```python
from build123d import *

# Parameters (mm, degrees)
CLIP_DEPTH        = 20.32
BACK_DEPTH        = 40.64
HOLE_DEPTH        = 6.08
COUNTERBORE_DEPTH = 1.397
CHAMFER1_SIZE     = 1.27
CHAMFER2_SIZE     = 0.508


with BuildPart() as part:
    # Sketch1 → clip (new body)
    with BuildSketch(Plane.XY):
        with BuildLine():
            Line((-2.629601498, -9.813806395), (-1.80785103, -6.746991897))
            ThreePointArc((-1.80785103, -6.746991897), (0, 6.985), (1.80785103, -6.746991897))
            Line((1.80785103, -6.746991897), (2.629601498, -9.813806395))
            Line((2.629601498, -9.813806395), (5.929158287, -11.718806395))
            Line((5.929158287, -11.718806395), (7.453158287, -9.079160964))
            Line((7.453158287, -9.079160964), (5.96856706, -8.22203182))
            ThreePointArc((5.96856706, -8.22203182), (9.051691591, -4.614377459), (10.16, 0))
            Line((10.16, 0), (10.16, 12.7))
            Line((10.16, 12.7), (-10.16, 12.7))
            Line((-10.16, 12.7), (-10.16, 0))
            ThreePointArc((-10.16, 0), (-9.051691591, -4.614377459), (-5.96856706, -8.22203182))
            Line((-5.96856706, -8.22203182), (-7.453158287, -9.079160964))
            Line((-7.453158287, -9.079160964), (-5.929158287, -11.718806395))
            Line((-5.929158287, -11.718806395), (-2.629601498, -9.813806395))
        make_face()
    extrude(amount=CLIP_DEPTH)

    # Sketch1_3 → back (add)
    with BuildSketch(Plane.XY):
        with BuildLine():
            ThreePointArc((0, 10.16), (-3.592102448, 9.503809762), (-6.72020833, 7.62))
            Line((-6.72020833, 7.62), (0, 7.62))
            Line((0, 7.62), (0, 10.16))
        make_face()
        with BuildLine():
            Line((0, 7.62), (6.72020833, 7.62))
            ThreePointArc((6.72020833, 7.62), (3.592102448, 9.503809762), (0, 10.16))
            Line((0, 10.16), (0, 7.62))
        make_face()
        with BuildLine():
            Line((-10.16, 12.7), (-10.16, 7.62))
            Line((-10.16, 7.62), (-6.72020833, 7.62))
            ThreePointArc((-6.72020833, 7.62), (-3.592102448, 9.503809762), (0, 10.16))
            ThreePointArc((0, 10.16), (3.592102448, 9.503809762), (6.72020833, 7.62))
            Line((6.72020833, 7.62), (10.16, 7.62))
            Line((10.16, 7.62), (10.16, 12.7))
            Line((10.16, 12.7), (-10.16, 12.7))
        make_face()
    extrude(amount=BACK_DEPTH)

    # Sketch4 → hole (cut, through all)
    with BuildSketch(Plane.XZ.offset(-7.62)):
        with BuildLine():
            Line((0, 35.705704095), (-1.26186816, 34.822134497))
            ThreePointArc((-1.26186816, 34.822134497), (0, 30.82), (1.26186816, 34.822134497))
            Line((1.26186816, 34.822134497), (0, 35.705704095))
        make_face()
    extrude(amount=-HOLE_DEPTH, mode=Mode.SUBTRACT)

    # Sketch4_3 → counterbore (cut)
    with BuildSketch(Plane.XZ.offset(-7.62)):
        with BuildLine():
            Line((0, 38.055695179), (-2.3660028, 36.399002183))
            ThreePointArc((-2.3660028, 36.399002183), (0, 28.895), (2.3660028, 36.399002183))
            Line((2.3660028, 36.399002183), (0, 38.055695179))
        make_face()
        with BuildLine():
            Line((-1.26186816, 34.822134497), (0, 35.705704095))
            Line((0, 35.705704095), (1.26186816, 34.822134497))
            ThreePointArc((1.26186816, 34.822134497), (0, 30.82), (-1.26186816, 34.822134497))
        make_face(mode=Mode.SUBTRACT)
    extrude(amount=-COUNTERBORE_DEPTH, mode=Mode.SUBTRACT)

    # Chamfer1
    chamfer1_edges = [part.edges().sort_by_distance(p)[0] for p in [
        (-10.16, 10.16, 40.64),
        (0, 7.62, 40.64),
        (10.16, 10.16, 40.64),
    ]]
    chamfer(chamfer1_edges, length=CHAMFER1_SIZE)

    # Chamfer2
    chamfer2_edges = [part.edges().sort_by_distance(p)[0] for p in [
        (7.453158287, -9.079160964, 10.16),
        (5.929158287, -11.718806395, 10.16),
        (-5.929158287, -11.718806395, 10.16),
        (-7.453158287, -9.079160964, 10.16),
        (-6.691158287, -10.39898368, 20.32),
        (6.691158287, -10.39898368, 20.32),
    ]]
    chamfer(chamfer2_edges, length=CHAMFER2_SIZE)


solid = part.part
```
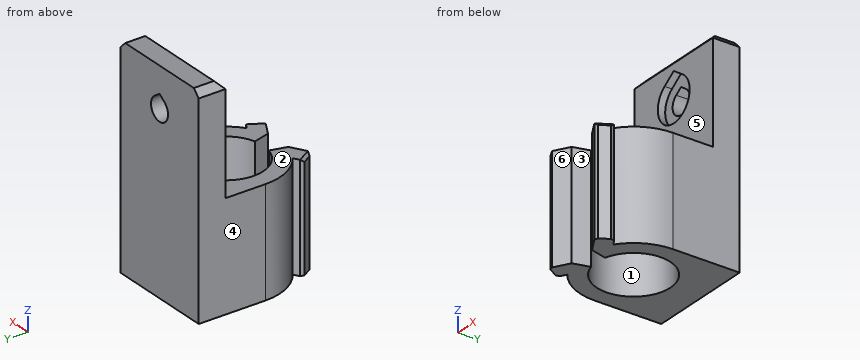
For this review, take the finished solid that the model builds, in its own axes (mm). Face numbers are marked on the shaded views. A direction names the side the tool comes from. Give positions to 0.01 mm unless a question says otherwise; leave off trailing zeros. Order: outer loops, then holes, each group sorted by start corner. A loop starts at its lowest first (then second) coordinate and runs counter-clockwise, first axis right, second up.
1) Take a section at C-C (y = -3). Give the boundary of the cut face in (x, z).
2) Take a section at D-D (x = -8). Give the boundary of the cut face in (y, z).
3) Take a section at A-A (z = 33.02). Give the boundary of the cut face in (x, y) (3 decimals), then the cut area to 3 significant figures.
4) Insertion check: pin 1 (7.5 mm diameter, centred on x = 0, z = 33.02, fed in from -Y); pin 2 (6.5 mm diameter, centred on x = 1.5, z = 32, fed in from -Y). Each pin has a flat end and moves straight along its axis. Give the tip position at first contact, or say it passes through.
5) The part is to be moulded in two halves that separate along Y. For the marked faces 1, 2 and 3, say which applies: released by +Y, released by -Y, zero draft, split by the parting line, or undercut.
6) Wall thickness on line 1 (X direction, y = 8.35, z = 33.02) (3 decimals); line 2 (Y direction, x = -5.75, z = 24.5); line 3 (X direction, y = 11.7, z = 33.02): over which ranges is each line inside the solid? List them lowest first.
7) Take a section at B-B (x = 4.75). Give the boundary of the cut face in (y, z), then the cut area to 3 significant figures.
8) For the marked faces 4, 5 and 6, list the 3-axis set-ups (+Z, -Z, +X, -X, +Y, -Y) from which the entire face can be reached by the end or side of a thin tool; tool diameter is ignored.
Derived:
1. outline: (-9.71, 0) - (-6.31, 0) - (-6.31, 20.32) - (-9.71, 20.32) - close; (6.31, 0) - (9.71, 0) - (9.71, 20.32) - (6.31, 20.32) - close
2. outline: (-6.26, 0) - (12.7, 0) - (12.7, 40.64) - (8.89, 40.64) - (7.62, 39.37) - (7.62, 20.32) - (-6.26, 20.32) - close
3. outline: (-10.16, 7.62) - (-4.125, 7.62) - (-4.125, 9.017) - (-2.2, 9.017) - (-2.2, 12.7) - (-10.16, 12.7) - close; (2.2, 9.017) - (4.125, 9.017) - (4.125, 7.62) - (10.16, 7.62) - (10.16, 12.7) - (2.2, 12.7) - close
3. area: 75.5 mm2
4. pin 1: stops at y = 9.02
4. pin 2: stops at y = 7.62
5. face 1: undercut
5. face 2: zero draft
5. face 3: released by -Y
6. line 1: x = -10.16 to -4.125, 4.125 to 10.16
6. line 2: y = 7.62 to 12.7
6. line 3: x = -10.16 to -2.2, 2.2 to 10.16
7. outline: (-11.04, 0) - (-5.12, 0) - (-5.12, 20.32) - (-11.04, 20.32) - close; (5.12, 0) - (12.7, 0) - (12.7, 40.64) - (8.89, 40.64) - (7.62, 39.37) - (7.62, 20.32) - (5.12, 20.32) - close
7. area: 377 mm2
8. face 4: +Z, -Z, -X, +Y, -Y
8. face 5: +Z, +X, -X, -Y
8. face 6: +Z, -Z, -Y
